```python
from build123d import *

# Parameters (mm, degrees)
SKETCH_1_R      = 6.5
EXTRUDE_1_DEPTH = 0.9
SKETCH_2_R      = 2
EXTRUDE_2_DEPTH = 10.15
SKETCH_3_R      = 6.5
EXTRUDE_3_DEPTH = 1.05
M2X0_4_1_D      = 1.6
M2X0_4_1_DEPTH  = 5.2
M2X0_4_1_TIP    = 0.480688495


with BuildPart() as part:
    # 草图1 → 凸台-拉伸1 (new body)
    with BuildSketch(Plane(origin=(0, 0, 0), x_dir=(1, 0, 0), z_dir=(0, 1, 0))):
        with Locations(Location((0, 0, 0), (0, 0, 270))):
            Circle(SKETCH_1_R)
    extrude(amount=EXTRUDE_1_DEPTH)

    # 草图2 → 凸台-拉伸2 (add)
    with BuildSketch(Plane(origin=(0, 0.9, 0), x_dir=(1, 0, 0), z_dir=(0, 1, 0))):
        with Locations(Location((0, 0, 0), (0, 0, 270))):
            Circle(SKETCH_2_R)
    extrude(amount=EXTRUDE_2_DEPTH)

    # 草图3 → 凸台-拉伸3 (add)
    with BuildSketch(Plane(origin=(0, 11.05, 0), x_dir=(1, 0, 0), z_dir=(0, 1, 0))):
        with Locations(Location((0, 0, 0), (0, 0, 270))):
            Circle(SKETCH_3_R)
    extrude(amount=EXTRUDE_3_DEPTH)

    # M2x0.4 螺纹孔1
    with Locations(Plane(origin=(0, 0, 0), x_dir=(0, 0, -1), z_dir=(0, -1, 0))):
        with Locations((0, 0)):
            Hole(M2X0_4_1_D / 2, depth=M2X0_4_1_DEPTH)
            with Locations((0, 0, -(M2X0_4_1_DEPTH + M2X0_4_1_TIP / 2))):  # 118° drill point
                Cone(0, M2X0_4_1_D / 2, M2X0_4_1_TIP, mode=Mode.SUBTRACT)


solid = part.part
```
For this review, take the finished solid that the model builds, in its own axes (mm). A direction names the side the tool comes from. Coordinates: 2 decimals unless noted, no trailing zeros. Loops run counter-clockwise (first coordinate to the right, second up) from the corner with the lowest first, then second, coordinate; pieces in that order, holes last.
1. For line 1 (Y direction, x = 4, z = -3.75); line 2 (X direction, y = 3.9, z = 0); line 3 (X direction, y = 7.25, z = 0), list the stretches that pass through material, from the lowest coordinate up.
2. Mouldability with a two-part tool opening along Y and no side actions: class faces 3 (the conical face through (0.006, 5.597, 0.139)), 4 (the flat face through (2, 11.05, 1)), 5 (the cylindrical face through (-0.49, 2.64, -0.63)) as +Y half, -Y half, draft (parallel to the pull), parting line (faces both ways), or undercut.
3. Add section C-C, the plane y = 9. Give the boundary of the cut face in (x, z).
4. Insertion check: P1, Ø1.5, axis at x = -2.5, y = 7.5, coming from the +Z side; P2, Ø5, axis at x = -1, y = 8, coming from the -Z side; P3, Ø6, axis at y = 10, z = 3.5, coming from the -X side. Each pin has a flat end and moves straight along its axis. Give the tip position at first contact, or say it passes through.
5. Add section A-A, the plane x = 5.75. Give the boundary of the cut face in (y, z).
6. Add section B-B, the plane z = 3.25. Give the boundary of the cut face in (x, y), then the cut area to 3 significant figures.
7. Add section D-D, the plane z = -1.5. Give the boundary of the cut face in (x, y), then the cut area to 3 significant figures.
8. For faces 1 (the cylindrical face through (-2, 6, 0)), 2 (the cylindrical face through (-3.955, 0.444, -5.158)), list the 3-axis set-ups (+Z, -Z, +X, -X, +Y, -Y) from which the entire face can be reached by the end or side of a thin tool; tool diameter is ignored.
Result:
1. line 1: y = 0 to 0.9, 11.05 to 12.1
1. line 2: x = -2 to -0.8, 0.8 to 2
1. line 3: x = -2 to 2
2. face 3: -Y half
2. face 4: undercut
2. face 5: draft
3. outline: circle Ø4 at (0, 0)
4. P1: stops at z = 0.97
4. P2: stops at z = -2
4. P3: stops at x = -6.46
5. outline: (0, -3.03) - (0.9, -3.03) - (0.9, 3.03) - (0, 3.03) - close; (11.05, -3.03) - (12.1, -3.03) - (12.1, 3.03) - (11.05, 3.03) - close
6. outline: (-5.63, 0) - (5.63, 0) - (5.63, 0.9) - (-5.63, 0.9) - close; (-5.63, 11.05) - (5.63, 11.05) - (5.63, 12.1) - (-5.63, 12.1) - close
6. area: 22.0 mm2
7. outline: (-6.32, 0) - (6.32, 0) - (6.32, 0.9) - (1.32, 0.9) - (1.32, 11.05) - (6.32, 11.05) - (6.32, 12.1) - (-6.32, 12.1) - (-6.32, 11.05) - (-1.32, 11.05) - (-1.32, 0.9) - (-6.32, 0.9) - close
7. area: 51.5 mm2
8. face 1: none
8. face 2: +Y, -Y
